from build123d import *

# Parameters (mm, degrees)
SKETCH1_W                                       = 200
SKETCH1_H                                       = 120
BOSS_EXTRUDE1_DEPTH                             = 3
CSK_FOR_M3_FLAT_HEAD_MACHINE_SCREW1_D           = 3
CSK_FOR_M3_FLAT_HEAD_MACHINE_SCREW1_CSINK_D     = 6
CSK_FOR_M3_FLAT_HEAD_MACHINE_SCREW1_CSINK_ANGLE = 90
FILLET1_R                                       = 8
BOSS_EXTRUDE2_DEPTH                             = 3
SKETCH9_R                                       = 2
CUT_EXTRUDE1_DEPTH                              = 4


with BuildPart() as part:
    # Sketch1 → Boss-Extrude1 (new body)
    with BuildSketch(Plane(origin=(0, 0, 0), x_dir=(1, 0, 0), z_dir=(0, 1, 0))):
        Rectangle(SKETCH1_W, SKETCH1_H)
    extrude(amount=BOSS_EXTRUDE1_DEPTH)

    # CSK for M3 Flat Head Machine Screw1 (through all)
    with Locations(Plane(origin=(0, 3, 0), x_dir=(1, 0, 0), z_dir=(0, 1, 0))):
        with Locations((-94, 54), (0, 54), (94, 54), (94, 0), (94, -54), (0, -54), (-94, -54), (-94, 0)):
            CounterSinkHole(CSK_FOR_M3_FLAT_HEAD_MACHINE_SCREW1_D / 2, CSK_FOR_M3_FLAT_HEAD_MACHINE_SCREW1_CSINK_D / 2, counter_sink_angle=CSK_FOR_M3_FLAT_HEAD_MACHINE_SCREW1_CSINK_ANGLE)

    # Fillet1
    fillet1_edges = [part.edges().sort_by_distance(p)[0] for p in [
        (100, 1.5, 60),
        (-100, 1.5, 60),
        (-100, 1.5, -60),
        (100, 1.5, -60),
    ]]
    fillet(fillet1_edges, radius=FILLET1_R)

    # Sketch7 → Boss-Extrude2 (add)
    with BuildSketch(Plane.XZ):
        with BuildLine():
            Line((100, 4), (103, 4))
            ThreePointArc((103, 4), (107, 0), (103, -4))
            Line((103, -4), (100, -4))
            Line((100, -4), (100, 4))
        make_face()
        with BuildLine():
            Line((-100, -4), (-103, -4))
            ThreePointArc((-103, -4), (-107, 0), (-103, 4))
            Line((-103, 4), (-100, 4))
            Line((-100, 4), (-100, -4))
        make_face()
    extrude(amount=-BOSS_EXTRUDE2_DEPTH)

    # Sketch9 → Cut-Extrude1 (cut)
    with BuildSketch(Plane(origin=(0, 3, 0), x_dir=(1, 0, 0), z_dir=(0, 1, 0))):
        with Locations(Location((-103, 0, 0), (0, 0, 270))):
            Circle(SKETCH9_R)
        with Locations(Location((103, 0, 0), (0, 0, 270))):
            Circle(SKETCH9_R)
    extrude(amount=-CUT_EXTRUDE1_DEPTH, mode=Mode.SUBTRACT)


solid = part.part
Could you check a few things on this model? Use its own coordinates, in mm. Give positions to 0.01 mm unless a question says otherwise; leave off trailing zeros. Order: outer loops, then holes, each group sorted by start corner. A loop starts at its lowest first (then second) coordinate and runs counter-clockwise, first axis right, second up. Notation, with made-up numbers: (-4, -30.75) -> (36, -30.75) arc R36 cw to (36, 6.25) -> close; hole circle Ø5 at (27, -28.5). An arc over 180 degrees is marked (long way). Answer in a Markdown table with one row per item. Add a question column.
Item 1: Please list where these lines run through material, in increasing order: probe 1 along Z at (x, y) = (0, 0.55); probe 2 along X at (y, z) = (1.1, -54); probe 3 along X at (y, z) = (2.8, 13.5).
Item 2: I'm going to push flat-ended pins straight in: P1, Ø1.5, axis at y = 1, z = 38.5, coming from the -X side; P2, Ø5, axis at x = -94, z = 54, coming from the +Y side; P3, Ø2.5, axis at x = 0, z = -54, coming from the +Y side; P4, Ø3.5, axis at x = -94, z = -54, coming from the -Y side. Where does each tip first touch, or does it pass through?
Item 3: Imagine slicing it at A-A (y = 0.45). Count the separate pieces of the cut face and the enclosed holes in it, and give its area (3 significant figures).
Item 4: We'd pull the mould along X, two halves only. Please class faces 1 (the cylindrical face through (-101, 2, 0)), 2 (the cylindrical face through (97.719, 1.521, -57.594)), 3 (the flat face through (-1, 0, -1)): pulls with the +X half, pulls with the -X half, needs draft (parallel to the pull), parting line crosses it, or undercut.
Item 5: Imagine slicing it at B-B (z = -33). List the corners of the cut face in (x, y) for me.
Result:
| question | item | result |
|---|---|---|
| 1 | probe 1 | -60 to -55.5, -52.5 to 52.5, 55.5 to 60 |
| 1 | probe 2 | -99.75 to -95.5, -92.5 to -1.5, 1.5 to 92.5, 95.5 to 99.75 |
| 1 | probe 3 | -100 to 100 |
| 2 | P1 | x = -100 |
| 2 | P2 | y = 2.5 |
| 2 | P3 | through |
| 2 | P4 | y = 0 |
| 3 | separate pieces | 1 |
| 3 | enclosed holes | 10 |
| 3 | area | 24,000 mm2 |
| 4 | face 1 | undercut |
| 4 | face 2 | pulls with the +X half |
| 4 | face 3 | needs draft |
| 5 | outline | (-100, 0) -> (100, 0) -> (100, 3) -> (-100, 3) -> close |
